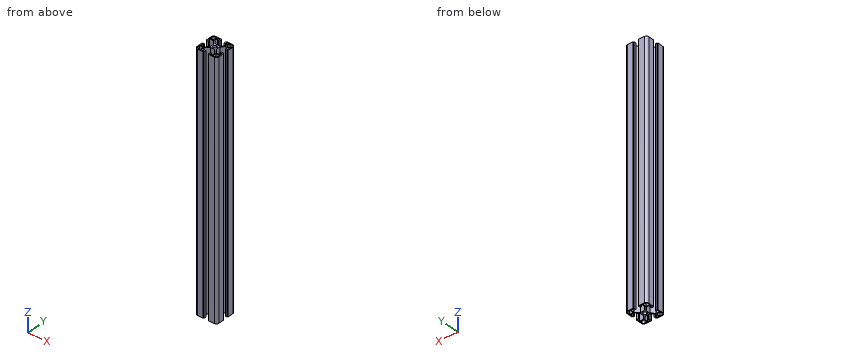
from build123d import *

# Parameters (mm, degrees)
BOSS_EXTRUDE1_DEPTH  = 460
MIRROR3_COPY_1_DEPTH = 460
MIRROR3_COPY_2_DEPTH = 460


with BuildPart() as part:
    # Sketch1 → Boss-Extrude1 (new body)
    with BuildSketch(Plane.XY):
        with BuildLine():
            Line((3.4, 0), (5.5, 0))
            Line((5.5, 0), (5.5, 4))
            Line((5.5, 4), (11.69, 10.19))
            Line((11.69, 10.19), (18.2, 10.19))
            Line((18.2, 10.19), (18.2, 6.3))
            Line((18.2, 6.3), (15.5, 6.3))
            Line((15.5, 6.3), (15.5, 4))
            Line((15.5, 4), (19, 4))
            Line((19, 4), (19, 5))
            Line((19, 5), (20, 5))
            Line((20, 5), (20, 15.5))
            ThreePointArc((20, 15.5), (18.681980515, 18.681980515), (15.5, 20))
            Line((15.5, 20), (5, 20))
            Line((5, 20), (5, 19))
            Line((5, 19), (4, 19))
            Line((4, 19), (4, 15.5))
            Line((4, 15.5), (6.3, 15.5))
            Line((6.3, 15.5), (6.3, 18.2))
            Line((6.3, 18.2), (10.19, 18.2))
            Line((10.19, 18.2), (10.19, 11.69))
            Line((10.19, 11.69), (4, 5.5))
            Line((4, 5.5), (0, 5.5))
            Line((0, 5.5), (0, 3.4))
            ThreePointArc((0, 3.4), (2.404163056, 2.404163056), (3.4, 0))
        make_face()
        with BuildLine():
            Line((18.5, 11.69), (18.5, 15.5))
            ThreePointArc((18.5, 15.5), (17.621320344, 17.621320344), (15.5, 18.5))
            Line((15.5, 18.5), (11.69, 18.5))
            Line((11.69, 18.5), (11.69, 11.69))
            Line((11.69, 11.69), (18.5, 11.69))
        make_face(mode=Mode.SUBTRACT)
    boss_extrude1 = extrude(amount=BOSS_EXTRUDE1_DEPTH)

    # Mirror1: Boss-Extrude1 across plane
    add(boss_extrude1.mirror(Plane.ZX))

    # Mirror2: Boss-Extrude1 across plane
    add(boss_extrude1.mirror(Plane(origin=(0, 0, 0), x_dir=(0, 0, 1), z_dir=(1, 0, 0))))

    # Mirror3 copy 1 sketch → Mirror3 copy 1 (add)
    with BuildSketch(Plane(origin=(0, 0, 0), x_dir=(-1, 0, 0), z_dir=(0, 0, 1))):
        with BuildLine():
            Line((3.4, 0), (5.5, 0))
            Line((5.5, 0), (5.5, 4))
            Line((5.5, 4), (11.69, 10.19))
            Line((11.69, 10.19), (18.2, 10.19))
            Line((18.2, 10.19), (18.2, 6.3))
            Line((18.2, 6.3), (15.5, 6.3))
            Line((15.5, 6.3), (15.5, 4))
            Line((15.5, 4), (19, 4))
            Line((19, 4), (19, 5))
            Line((19, 5), (20, 5))
            Line((20, 5), (20, 15.5))
            ThreePointArc((20, 15.5), (18.681980515, 18.681980515), (15.5, 20))
            Line((15.5, 20), (5, 20))
            Line((5, 20), (5, 19))
            Line((5, 19), (4, 19))
            Line((4, 19), (4, 15.5))
            Line((4, 15.5), (6.3, 15.5))
            Line((6.3, 15.5), (6.3, 18.2))
            Line((6.3, 18.2), (10.19, 18.2))
            Line((10.19, 18.2), (10.19, 11.69))
            Line((10.19, 11.69), (4, 5.5))
            Line((4, 5.5), (0, 5.5))
            Line((0, 5.5), (0, 3.4))
            ThreePointArc((0, 3.4), (2.404163056, 2.404163056), (3.4, 0))
        make_face()
        with BuildLine():
            Line((18.5, 11.69), (18.5, 15.5))
            ThreePointArc((18.5, 15.5), (17.621320344, 17.621320344), (15.5, 18.5))
            Line((15.5, 18.5), (11.69, 18.5))
            Line((11.69, 18.5), (11.69, 11.69))
            Line((11.69, 11.69), (18.5, 11.69))
        make_face(mode=Mode.SUBTRACT)
    extrude(amount=MIRROR3_COPY_1_DEPTH)

    # Mirror3 copy 2 sketch → Mirror3 copy 2 (add)
    with BuildSketch(Plane.XY):
        with BuildLine():
            Line((3.4, 0), (5.5, 0))
            Line((5.5, 0), (5.5, -4))
            Line((5.5, -4), (11.69, -10.19))
            Line((11.69, -10.19), (18.2, -10.19))
            Line((18.2, -10.19), (18.2, -6.3))
            Line((18.2, -6.3), (15.5, -6.3))
            Line((15.5, -6.3), (15.5, -4))
            Line((15.5, -4), (19, -4))
            Line((19, -4), (19, -5))
            Line((19, -5), (20, -5))
            Line((20, -5), (20, -15.5))
            ThreePointArc((20, -15.5), (18.681980515, -18.681980515), (15.5, -20))
            Line((15.5, -20), (5, -20))
            Line((5, -20), (5, -19))
            Line((5, -19), (4, -19))
            Line((4, -19), (4, -15.5))
            Line((4, -15.5), (6.3, -15.5))
            Line((6.3, -15.5), (6.3, -18.2))
            Line((6.3, -18.2), (10.19, -18.2))
            Line((10.19, -18.2), (10.19, -11.69))
            Line((10.19, -11.69), (4, -5.5))
            Line((4, -5.5), (0, -5.5))
            Line((0, -5.5), (0, -3.4))
            ThreePointArc((0, -3.4), (2.404163056, -2.404163056), (3.4, 0))
        make_face()
        with BuildLine():
            Line((18.5, -11.69), (18.5, -15.5))
            ThreePointArc((18.5, -15.5), (17.621320344, -17.621320344), (15.5, -18.5))
            Line((15.5, -18.5), (11.69, -18.5))
            Line((11.69, -18.5), (11.69, -11.69))
            Line((11.69, -11.69), (18.5, -11.69))
        make_face(mode=Mode.SUBTRACT)
    extrude(amount=MIRROR3_COPY_2_DEPTH)


solid = part.part
Build history of the part. All positions in model axes, mm. Give positions to 0.01 mm unless a question says otherwise; leave off trailing zeros. Put each result on its own line as item: value.
Item 1: Cut at A-A on z = 204.5. Count the separate pieces of the cut face and the enclosed holes in it, then the cut area to 3 significant figures.
Results are:
separate pieces: 1
enclosed holes: 5
area: 471 mm2
Item 2: Wall check: probe 1 along X at (y, z) = (-13, 25.5); probe 2 along Y at (x, z) = (7, 333.5). Give the ranges that are in metal, low to high.
Results are:
probe 1: -20 to -18.5, -11.69 to -10.19, 10.19 to 11.69, 18.5 to 20
probe 2: -20 to -18.2, -8.5 to -5.5, 5.5 to 8.5, 18.2 to 20
Item 3: Drop flat-ended pins along their axis: pin 1 Ø6.5 at (y, z) = (-1.5, 227) entering from -X; pin 2 Ø0.8 at (x, z) = (-4.5, 185.5) entering from -Y; pin 3 Ø1 at (x, y) = (8, -11.5) entering from -Z; pin 4 Ø4 at (x, z) = (-18, 177) entering from +Y. Give the stop position or say it passes through.
Results are:
pin 1: x = -19
pin 2: y = -19
pin 3: through
pin 4: y = 19.97
